The listing builds one solid part. Answer for the finished solid, in the listing's coordinates (mm). Coordinates: 2 decimals unless noted, no trailing zeros. Order: outer loops, then holes, each group sorted by start corner. A loop starts at its lowest first (then second) coordinate and runs counter-clockwise, first axis right, second up.
from build123d import *

# Parameters (mm, degrees)
SKETCH_2_R      = 145.099960032
EXTRUDE_1_DEPTH = 30


with BuildPart() as part:
    # 草圖2 → 填料-伸長1 (new body)
    with BuildSketch(Plane(origin=(0, 0, 0), x_dir=(1, 0, 0), z_dir=(0, 1, 0))):
        with Locations(Location((0, 0, 0), (0, 0, 270))):
            Circle(SKETCH_2_R)
        with BuildLine():
            Line((29.2365868, 106.161301764), (33.871841715, 120.427149509))
            ThreePointArc((33.871841715, 120.427149509), (19.569945324, 123.559771932), (5, 125))
            Line((5, 125), (5, 110))
            Line((5, 110), (-5, 110))
            Line((-5, 110), (-5, 125))
            ThreePointArc((-5, 125), (-19.569945324, 123.559771932), (-33.871841715, 120.427149509))
            Line((-33.871841715, 120.427149509), (-29.2365868, 106.161301764))
            Line((-29.2365868, 106.161301764), (-38.747151963, 103.071131821))
            Line((-38.747151963, 103.071131821), (-43.382406878, 117.336979565))
            ThreePointArc((-43.382406878, 117.336979565), (-56.794193372, 111.464880564), (-69.428071565, 104.066050558))
            Line((-69.428071565, 104.066050558), (-60.61129278, 91.930795643))
            Line((-60.61129278, 91.930795643), (-68.701462724, 86.05294312))
            Line((-68.701462724, 86.05294312), (-77.518241508, 98.188198035))
            ThreePointArc((-77.518241508, 98.188198035), (-88.459030065, 88.459030065), (-98.188198035, 77.518241508))
            Line((-98.188198035, 77.518241508), (-86.05294312, 68.701462724))
            Line((-86.05294312, 68.701462724), (-91.930795643, 60.61129278))
            Line((-91.930795643, 60.61129278), (-104.066050558, 69.428071565))
            ThreePointArc((-104.066050558, 69.428071565), (-111.464880564, 56.794193372), (-117.336979565, 43.382406878))
            Line((-117.336979565, 43.382406878), (-103.071131821, 38.747151963))
            Line((-103.071131821, 38.747151963), (-106.161301764, 29.2365868))
            Line((-106.161301764, 29.2365868), (-120.427149509, 33.871841715))
            ThreePointArc((-120.427149509, 33.871841715), (-123.559771932, 19.569945324), (-125, 5))
            Line((-125, 5), (-110, 5))
            Line((-110, 5), (-110, -5))
            Line((-110, -5), (-125, -5))
            ThreePointArc((-125, -5), (-123.559771932, -19.569945324), (-120.427149509, -33.871841715))
            Line((-120.427149509, -33.871841715), (-106.161301764, -29.2365868))
            Line((-106.161301764, -29.2365868), (-103.071131821, -38.747151963))
            Line((-103.071131821, -38.747151963), (-117.336979565, -43.382406878))
            ThreePointArc((-117.336979565, -43.382406878), (-111.464880564, -56.794193372), (-104.066050558, -69.428071565))
            Line((-104.066050558, -69.428071565), (-91.930795643, -60.61129278))
            Line((-91.930795643, -60.61129278), (-86.05294312, -68.701462724))
            Line((-86.05294312, -68.701462724), (-98.188198035, -77.518241508))
            ThreePointArc((-98.188198035, -77.518241508), (-88.459030065, -88.459030065), (-77.518241508, -98.188198035))
            Line((-77.518241508, -98.188198035), (-68.701462724, -86.05294312))
            Line((-68.701462724, -86.05294312), (-60.61129278, -91.930795643))
            Line((-60.61129278, -91.930795643), (-69.428071565, -104.066050558))
            ThreePointArc((-69.428071565, -104.066050558), (-56.794193372, -111.464880564), (-43.382406878, -117.336979565))
            Line((-43.382406878, -117.336979565), (-38.747151963, -103.071131821))
            Line((-38.747151963, -103.071131821), (-29.2365868, -106.161301764))
            Line((-29.2365868, -106.161301764), (-33.871841715, -120.427149509))
            ThreePointArc((-33.871841715, -120.427149509), (-19.569945324, -123.559771932), (-5, -125))
            Line((-5, -125), (-5, -110))
            Line((-5, -110), (5, -110))
            Line((5, -110), (5, -125))
            ThreePointArc((5, -125), (19.569945324, -123.559771932), (33.871841715, -120.427149509))
            Line((33.871841715, -120.427149509), (29.2365868, -106.161301764))
            Line((29.2365868, -106.161301764), (38.747151963, -103.071131821))
            Line((38.747151963, -103.071131821), (43.382406878, -117.336979565))
            ThreePointArc((43.382406878, -117.336979565), (56.794193372, -111.464880564), (69.428071565, -104.066050558))
            Line((69.428071565, -104.066050558), (60.61129278, -91.930795643))
            Line((60.61129278, -91.930795643), (68.701462724, -86.05294312))
            Line((68.701462724, -86.05294312), (77.518241508, -98.188198035))
            ThreePointArc((77.518241508, -98.188198035), (88.459030065, -88.459030065), (98.188198035, -77.518241508))
            Line((98.188198035, -77.518241508), (86.05294312, -68.701462724))
            Line((86.05294312, -68.701462724), (91.930795643, -60.61129278))
            Line((91.930795643, -60.61129278), (104.066050558, -69.428071565))
            ThreePointArc((104.066050558, -69.428071565), (111.464880564, -56.794193372), (117.336979565, -43.382406878))
            Line((117.336979565, -43.382406878), (103.071131821, -38.747151963))
            Line((103.071131821, -38.747151963), (106.161301764, -29.2365868))
            Line((106.161301764, -29.2365868), (120.427149509, -33.871841715))
            ThreePointArc((120.427149509, -33.871841715), (123.559771932, -19.569945324), (125, -5))
            Line((125, -5), (110, -5))
            Line((110, -5), (110, 5))
            Line((110, 5), (125, 5))
            ThreePointArc((125, 5), (123.559771932, 19.569945324), (120.427149509, 33.871841715))
            Line((120.427149509, 33.871841715), (106.161301764, 29.2365868))
            Line((106.161301764, 29.2365868), (103.071131821, 38.747151963))
            Line((103.071131821, 38.747151963), (117.336979565, 43.382406878))
            ThreePointArc((117.336979565, 43.382406878), (111.464880564, 56.794193372), (104.066050558, 69.428071565))
            Line((104.066050558, 69.428071565), (91.930795643, 60.61129278))
            Line((91.930795643, 60.61129278), (86.05294312, 68.701462724))
            Line((86.05294312, 68.701462724), (98.188198035, 77.518241508))
            ThreePointArc((98.188198035, 77.518241508), (88.459030065, 88.459030065), (77.518241508, 98.188198035))
            Line((77.518241508, 98.188198035), (68.701462724, 86.05294312))
            Line((68.701462724, 86.05294312), (60.61129278, 91.930795643))
            Line((60.61129278, 91.930795643), (69.428071565, 104.066050558))
            ThreePointArc((69.428071565, 104.066050558), (56.794193372, 111.464880564), (43.382406878, 117.336979565))
            Line((43.382406878, 117.336979565), (38.747151963, 103.071131821))
            Line((38.747151963, 103.071131821), (29.2365868, 106.161301764))
        make_face(mode=Mode.SUBTRACT)
    extrude(amount=EXTRUDE_1_DEPTH)


solid = part.part
1) Consider L1, parallel to X at y = 16.25, z = 119.5; L2, parallel to Z at x = -113.5, y = 24.5; L3, parallel to Z at x = -106.5, y = 14.25. Determine where each line is inside the solid, lowest interval first.
2) Section A-A (z = 0) is taken. Give the vertices of the cut face in (x, y), then the cut area to 3 significant figures.
3) Determine the mould class of faces 1 (the face through (43.58, 14.79, 138.4)), 2 (the face through (19.772, 14.79, -123.528)) for opening direction X: released by +X, released by -X, zero draft, split by the parting line, or undercut.
4) Section B-B (x = 0) is taken. Give the vertices of the cut face in (y, z).
5) Each of these flat-tipped pins is pushed along its axis until it touches: P1, Ø12, axis at y = 9, z = -114.5, coming from the -X side; P2, Ø4.5, axis at y = 15.5, z = -118, coming from the +X side; P3, Ø7.5, axis at x = -120.5, y = 14, coming from the -Z side. Where does it stop, or does it pass through?
Filled sheet:
1. L1: x = -82.3 to -33.57, -5 to 5, 33.57 to 82.3
1. L2: z = -90.4 to -52.61, -42.14 to -31.62, -5 to 5, 31.62 to 42.14, 52.61 to 90.4
1. L3: z = -98.55 to -65.63, -39.86 to -29.35, 29.35 to 39.86, 65.63 to 98.55
2. outline: (-145.1, 0) - (-110, 0) - (-110, 30) - (-145.1, 30) - close; (110, 0) - (145.1, 0) - (145.1, 30) - (110, 30) - close
2. area: 2,110 mm2
3. face 1: split by the parting line
3. face 2: undercut
4. outline: (0, -145.1) - (30, -145.1) - (30, -110) - (0, -110) - close; (0, 110) - (30, 110) - (30, 145.1) - (0, 145.1) - close
5. P1: stops at x = -96.34
5. P2: stops at x = 87.5
5. P3: stops at z = -86.16
